Autodesk Inventor part; units mm, degrees
ref_plane "YZ Plane" through (0, 0, 0) normal (1, 0, 0) x (0, 1, 0)
ref_plane "XZ Plane" through (0, 0, 0) normal (0, 1, 0) x (-1, 0, 0)
ref_plane "XY Plane" through (0, 0, 0) normal (0, 0, 1) x (1, 0, 0)
sketch "Sketch8" plane through (0, 0, 0) normal (0, 0, 1) x (1, 0, 0)
  line L0 (-23.4899, -4.07) -> (-4.7399, -4.07)
  line L1 (-4.7399, -4.07) -> (-4.7399, 10.93)
  line L2 (-4.7399, 10.93) -> (-23.4899, 10.93)
  line L3 (-23.4899, 10.93) -> (-23.4899, -4.07)
  line L4 (5.9, -21.53) -> (12.9, -21.53)
  line L5 (12.9, -21.53) -> (12.9, 21.53)
  line L6 (12.9, 21.53) -> (5.9, 21.53)
  line L7 (9.6, -27.93) -> (13.2, -27.93)
  line L8 (-21.4963, 16.93) -> (5.9, 16.93)
  line L9 (5.9, 16.93) -> (5.9, 27.93)
  line L10 (5.9, 27.93) -> (21.5, 27.93)
  line L11 (21.5, 27.93) -> (21.5, -27.93)
  line L12 (21.5, -27.93) -> (5.9, -27.93)
  line L13 (5.9, -27.93) -> (5.9, -18.57)
  line L14 (5.9, -18.57) -> (-21.4789, -18.57)
  line L15 (-21.4789, -18.57) -> (-32.4963, -18.57)
  line L16 (-32.4963, -18.57) -> (-32.4963, 16.93)
  line L17 (-32.4963, 16.93) -> (-21.4963, 16.93)
  point P0 (0, 0)
  point P1 (5.9, -27.93)
extrude "Extrusion10" add sketch "Sketch8" along normal blind 14 contours L4 L5 L6 L9 L10 L11 L12 L7 L13
extrude "Extrusion11" add sketch "Sketch8" along normal blind 13.2 contours L3 L2 L1 L0
extrude "Extrusion12" add sketch "Sketch8" along normal blind 5.8 contours L13 L14 L15 L16 L17 L8 L9 L6 L5 L4
properties part number "heatsink_2"
CAD build for the part. Positions are in the model's coordinates, mm. A direction names the side the tool comes from. Coordinates: 2 decimals unless noted, no trailing zeros. Write each loop counter-clockwise with the first axis right and the second up, starting at its lowest first coordinate (ties: lowest second). Pieces come first, ordered by that corner, then holes. Notation, with made-up numbers: M 63.25,62.5 L 109.25,62.5 A23 cw 109.25,76.5 Z; hole C -10.5,88 d8. An arc over 180 degrees is marked long. Answer as a JSON object with one key per item and string values. Group by question number.
1) Mould opens along X. For faces 1 (the face through (-4.74, 3, 9)), 2 (the face through (21.5, 0, 7)), 3 (the face through (-13, -18.57, 3)), 4 (the face through (-10.1, -4.5, 5.8)) say: +X half, -X half, draft (parallel to the pull), parting line (faces both ways), or undercut.
2) Wall check: line 1 (X direction, y = -8, z = 10.75); line 2 (Z direction, x = -5.5, y = 16.5); line 3 (Z direction, x = -8, y = 2). Give the ranges that are in metal, low to high. Write a range as from..to.
3) Tool access for faces 5 (the face through (5.9, -24, 7)), 6 (the face through (12.9, 0, 10)), 7 (the face through (-14, 16.93, 3)), 8 (the face through (-23.49, 4, 9)): list every direction of +Z, -Z, +X, -X, +Y, -Y with a clear straight run to the whole face (end or side of a thin tool).
4) Saw through at A-A (z = 10.75). Write the cut outline in (x, y), plus the area to 3 significant figures.
5) Pin check, flat tips, straight feed: pin 1 Ø1 at (x, y) = (-20.5, -13) entering from -Z; pin 2 Ø3.5 at (y, z) = (24.5, 5) entering from -X; pin 3 Ø13 at (x, y) = (-6, 4) entering from +Z; pin 4 Ø6 at (x, y) = (-8.5, -19) entering from +Z. Stop position of each tip, or through.
6) Saw through at D-D (z = 3). Write the cut outline in (x, y), plus the area to 3 significant figures.
7) Saw through at C-C (x = -13). Write the cut outline in (y, z).
8) Saw through at B-B (y = 5). Write the cut outline in (x, z).
Values follow:
{
 "1": {"face 1": "undercut", "face 2": "+X half", "face 3": "draft", "face 4": "undercut"},
 "2": {"line 1": "x = 12.9..21.5", "line 2": "z = 0..5.8", "line 3": "z = 0..13.2"},
 "3": {"face 5": "+Z, -Z, -X, -Y", "face 6": "+Z", "face 7": "+Z, -Z, -X, +Y", "face 8": "+Z, -X, +Y, -Y"},
 "4": {"outline": "M -23.49,-4.07 L -4.74,-4.07 L -4.74,10.93 L -23.49,10.93 Z; M 5.9,-27.93 L 21.5,-27.93 L 21.5,27.93 L 5.9,27.93 L 5.9,21.53 L 12.9,21.53 L 12.9,-21.53 L 5.9,-21.53 Z", "area": "851 mm2"},
 "5": {"pin 1": "stops at z = 0", "pin 2": "stops at x = 5.9", "pin 3": "stops at z = 13.2", "pin 4": "stops at z = 5.8"},
 "6": {"outline": "M -32.5,-18.57 L 5.9,-18.57 L 5.9,-27.93 L 21.5,-27.93 L 21.5,27.93 L 5.9,27.93 L 5.9,16.93 L -32.5,16.93 Z", "area": "2,230 mm2"},
 "7": {"outline": "M -18.57,0 L 16.93,0 L 16.93,5.8 L 10.93,5.8 L 10.93,13.2 L -4.07,13.2 L -4.07,5.8 L -18.57,5.8 Z"},
 "8": {"outline": "M -32.5,0 L 21.5,0 L 21.5,14 L 12.9,14 L 12.9,5.8 L -4.74,5.8 L -4.74,13.2 L -23.49,13.2 L -23.49,5.8 L -32.5,5.8 Z"}
}
